Geometry check sheet. Reference: drawing and pictorial views, mm from the part's lowest x, y, z. A direction names the side the tool comes from. Give positions to 0.01 mm unless a question says otherwise; leave off trailing zeros. Loops run counter-clockwise (first coordinate to the right, second up) from the corner with the lowest first, then second, coordinate; pieces in that order, holes last. Notation, with made-up numbers: (66, 50) - (93, 50) arc R21 cw to (93, 57) - close; hole circle Ø5 at (19, 51). An arc over 180 degrees is marked (long way). Use CSV: the item, a comma, the result in double quotes.
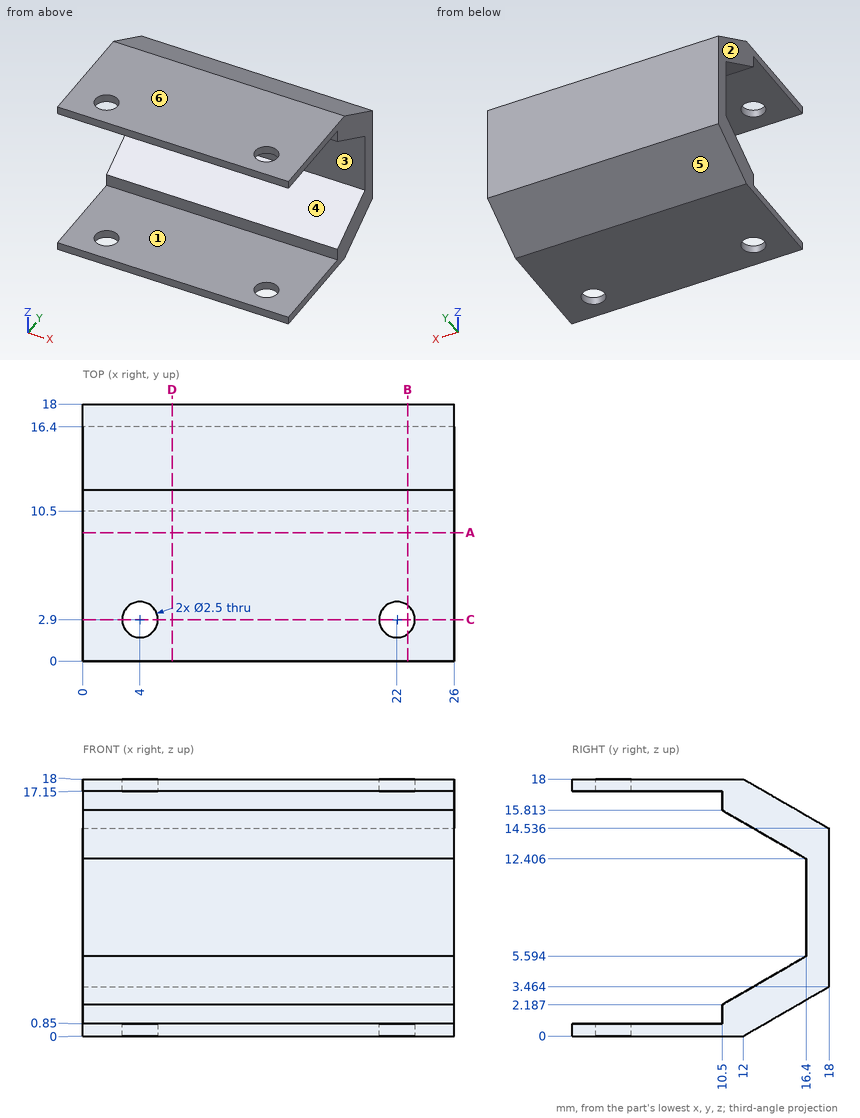
1. Sectioned sample at B-B, the plane x = 22.75. Record the boundary of the cut face in (y, z).
Completed:
outline,"(0, 0) - (1.9, 0) - (1.9, 0.85) - (0, 0.85) - close; (0, 17.15) - (1.9, 17.15) - (1.9, 18) - (0, 18) - close; (3.9, 0) - (12, 0) - (18, 3.46) - (18, 14.54) - (12, 18) - (3.9, 18) - (3.9, 17.15) - (10.5, 17.15) - (10.5, 15.81) - (16.4, 12.41) - (16.4, 5.59) - (10.5, 2.19) - (10.5, 0.85) - (3.9, 0.85) - close"
2. Sectioned sample at C-C, the plane y = 2.9. Record the boundary of the cut face in (x, z).
Completed:
outline,"(0, 0) - (2.75, 0) - (2.75, 0.85) - (0, 0.85) - close; (0, 17.15) - (2.75, 17.15) - (2.75, 18) - (0, 18) - close; (5.25, 0) - (20.75, 0) - (20.75, 0.85) - (5.25, 0.85) - close; (5.25, 17.15) - (20.75, 17.15) - (20.75, 18) - (5.25, 18) - close; (23.25, 0) - (26, 0) - (26, 0.85) - (23.25, 0.85) - close; (23.25, 17.15) - (26, 17.15) - (26, 18) - (23.25, 18) - close"
3. Sectioned sample at A-A, the plane y = 9. Record the boundary of the cut face in (x, z).
Completed:
outline,"(0, 0) - (26, 0) - (26, 0.85) - (0, 0.85) - close; (0, 17.15) - (26, 17.15) - (26, 18) - (0, 18) - close"
4. Release check for a two-part mould opening along Z. For the marked faces 3, 4, 5 and 6 record: released by +Z, released by -Z, zero draft, split by the parting line, or undercut.
Completed:
face 3,"undercut"
face 4,"undercut"
face 5,"released by -Z"
face 6,"released by +Z"
5. Set-up check for the marked faces 1 and 2: record each of +Z, -Z, +X, -X, +Y, -Y from which the full face is reachable in a straight line by a thin tool's end or side.
Completed:
face 1,"+X, -X, -Y"
face 2,"+Z, -Z, -X, +Y, -Y"
6. Scan lines: line 1 along Z through (x, y) = (7.25, 1); line 2 along Z through (x, y) = (4.5, 13.5) (1 decimal); line 3 along Y through (x, z) = (22, 0.6). Record each from-to range of solid material in increasing order.
Completed:
line 1,"z = 0 to 0.85, 17.15 to 18"
line 2,"z = 0.9 to 3.9, 14.1 to 17.1"
line 3,"y = 0 to 1.65, 4.15 to 13.04"
7. Sectioned sample at D-D, the plane x = 6.25. Record the boundary of the cut face in (y, z).
Completed:
outline,"(0, 0) - (12, 0) - (18, 3.46) - (18, 14.54) - (12, 18) - (0, 18) - (0, 17.15) - (10.5, 17.15) - (10.5, 15.81) - (16.4, 12.41) - (16.4, 5.59) - (10.5, 2.19) - (10.5, 0.85) - (0, 0.85) - close"
8. Go/stop test with flat-tipped pins: pin 1 Ø5 at (x, z) = (6.5, 5) entering from -Y; pin 2 Ø1.5 at (x, y) = (4, 2.9) entering from +Z; pin 3 Ø1 at (x, z) = (8, 13) entering from -Y (1 decimal); pin 4 Ø1.1 at (x, z) = (9, 16.5) entering from -Y. Record where each tip stops, or that it passes through.
Completed:
pin 1,"stops at y = 11.04"
pin 2,"passes through"
pin 3,"stops at y = 14.5"
pin 4,"stops at y = 10.5"
